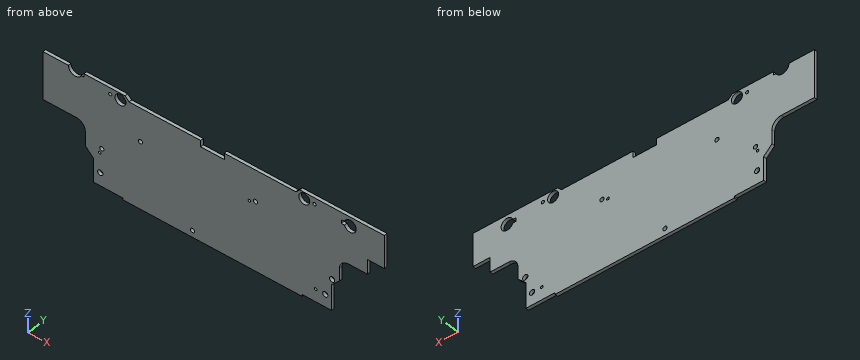
from build123d import *

# Parameters (mm, degrees)
BOSS_EXTRU_1_DEPTH      = 1.2
ESQUISSE1_4_R           = 2.1
ESQUISSE1_4_R_2         = 0.8
ESQUISSE1_4_R_3         = 1
ESQUISSE1_4_R_4         = 0.5
ESQUISSE1_4_R_5         = 0.6
ENL_V_MAT_EXTRU_1_DEPTH = 1.2


with BuildPart() as part:
    # Esquisse1 → Boss.-Extru.1 (new body)
    with BuildSketch(Plane(origin=(0, 0, 0), x_dir=(1, 0, 0), z_dir=(0, 1, 0))):
        with BuildLine():
            Line((-64.55, 14.3), (-64.55, -3.9))
            Line((-64.55, -3.9), (-54.85, -3.9))
            ThreePointArc((-54.85, -3.9), (-52.920836567, -1.286846787), (-49.95, -2.6))
            Line((-49.95, -2.6), (-48.95, -2.6))
            Line((-48.95, -2.6), (-48.95, -3.9))
            Line((-48.95, -3.9), (-33.25, -3.9))
            Line((-33.25, -3.9), (-31.75, -2.4))
            Line((-31.75, -2.4), (-4.5, -2.4))
            Line((-4.5, -2.4), (-4.5, 0))
            Line((-4.5, 0), (4.5, 0))
            Line((4.5, 0), (4.5, -2.4))
            Line((4.5, -2.4), (31.75, -2.4))
            Line((31.75, -2.4), (33.25, -3.9))
            Line((33.25, -3.9), (65.45, -3.9))
            Line((65.45, -3.9), (65.45, 8.7))
            Line((65.45, 8.7), (58.95, 8.7))
            Line((58.95, 8.7), (58.95, 14.3))
            Line((58.95, 14.3), (51.85, 14.3))
            ThreePointArc((51.85, 14.3), (49.375126266, 15.325126266), (48.35, 17.8))
            Line((48.35, 17.8), (48.35, 22.6))
            Line((48.35, 22.6), (45.35, 25.6))
            Line((45.35, 25.6), (45.35, 35.4))
            Line((45.35, 35.4), (34.15, 35.4))
            Line((34.15, 35.4), (34.15, 36.1))
            Line((34.15, 36.1), (-34.05, 36.1))
            Line((-34.05, 36.1), (-34.05, 35.4))
            Line((-34.05, 35.4), (-45.25, 35.4))
            Line((-45.25, 35.4), (-45.25, 26.4))
            Line((-45.25, 26.4), (-48.45, 23.2))
            Line((-48.45, 23.2), (-48.45, 17.8))
            ThreePointArc((-48.45, 17.8), (-49.475126266, 15.325126266), (-51.95, 14.3))
            Line((-51.95, 14.3), (-64.55, 14.3))
        make_face()
    extrude(amount=BOSS_EXTRU_1_DEPTH)

    # Esquisse1_4 → Enl_v. mat.-Extru.1 (cut)
    with BuildSketch(Plane(origin=(0, 0, 0), x_dir=(1, 0, 0), z_dir=(0, 1, 0))):
        with BuildLine():
            Line((49.05, -1.1), (50.25910977, -1.1))
            ThreePointArc((50.25910977, -1.1), (54.75, -0.4), (50.25910977, 0.3))
            Line((50.25910977, 0.3), (49.05, 0.3))
            Line((49.05, 0.3), (49.05, -1.1))
        make_face()
        with Locations((34.95, -1.4)):
            Circle(ESQUISSE1_4_R)
        with Locations((-35.05, -1.4)):
            Circle(ESQUISSE1_4_R)
        with Locations((-7.65, 33.5)):
            Circle(ESQUISSE1_4_R_2)
        with Locations((42.95, 30.6)):
            Circle(ESQUISSE1_4_R_3)
        with Locations((-27.45, 10.4)):
            Circle(ESQUISSE1_4_R_2)
        with Locations((16.35, 9.6)):
            Circle(ESQUISSE1_4_R_2)
        with Locations((-42.95, 22.9)):
            Circle(ESQUISSE1_4_R_4)
        with Locations((-42.75, 30.4)):
            Circle(ESQUISSE1_4_R_3)
        with Locations((45.55, 23.5)):
            Circle(ESQUISSE1_4_R_3)
        with Locations((14.05, 10.5)):
            Circle(ESQUISSE1_4_R_4)
        with Locations((-42.15, 21)):
            Circle(ESQUISSE1_4_R_2)
        with Locations((-38.95, -1.5)):
            Circle(ESQUISSE1_4_R_5)
        with Locations((39.25, 30.6)):
            Circle(ESQUISSE1_4_R_4)
        with Locations((38.85, -1.5)):
            Circle(ESQUISSE1_4_R_5)
    extrude(amount=ENL_V_MAT_EXTRU_1_DEPTH, mode=Mode.SUBTRACT)


solid = part.part
Here's how the part is built. I have some questions about the finished solid (model axes, mm). Round coordinates to 2 decimals unless told otherwise and drop trailing zeros. Order: outer loops, then holes, each group sorted by start corner. A loop starts at its lowest first (then second) coordinate and runs counter-clockwise, first axis right, second up. Notation, with made-up numbers: M -38.5,-36 L -27.5,-36 A24 cw -27.5,-7 Z; hole C -16,43.5 d8. An arc over 180 degrees is marked long. Return JSON: item names as keys, results as strings. Group by question number.
1. If we section it at C-C on x = -18: List the corners of the cut face in (y, z) for me.
2. Please list where these lines run through material, in increasing order: probe 1 along Z at (x, y) = (-35, 1.15); probe 2 along X at (y, z) = (0.6, -10.5); probe 3 along Z at (x, y) = (-38.95, 0.6).
3. I'm going to push flat-ended pins straight in: pin 1 Ø0.6 at (y, z) = (0.5, -31.5) entering from -X; pin 2 Ø0.6 at (x, y) = (37, 1) entering from -Z. Where does each tip first touch, or does it pass through?
4. If we section it at A-A on x = 35.5: List the corners of the cut face in (y, z) for me, then the cut area to 3 significant figures.
5. If we section it at B-B on y = 0.7: State how many separate pieces and enclosed holes the cut face has, then the cut area to 3 significant figures.
Reply:
{
 "1": {"outline": "M 0,-36.1 L 1.2,-36.1 L 1.2,2.4 L 0,2.4 Z"},
 "2": {"probe 1": "-35.4 to -0.7, 3.5 to 3.9", "probe 2": "-64.55 to -28.24, -26.66 to 13.55, 14.55 to 58.95", "probe 3": "-35.4 to 0.9, 2.1 to 3.9"},
 "3": {"pin 1": "x = -45.25", "pin 2": "z = -35.4"},
 "4": {"outline": "M 0,-35.4 L 1.2,-35.4 L 1.2,-0.63 L 0,-0.63 Z; M 0,3.43 L 1.2,3.43 L 1.2,3.9 L 0,3.9 Z", "area": "42.3 mm^2"},
 "5": {"separate pieces": "1", "enclosed holes": "15", "area": "4,160 mm^2"}
}
